```python
from build123d import *

# Parameters (mm, degrees)
SKETCH1_R           = 0.762
BOSS_EXTRUDE1_DEPTH = 0.381


with BuildPart() as part:
    # Sketch1 → Boss-Extrude1 (new, symmetric)
    with BuildSketch(Plane(origin=(0, 0, 0), x_dir=(1, 0, 0), z_dir=(0, 1, 0))):
        with BuildLine():
            Line((-0.172545192, 1.641958939), (1.605454808, 1.8288))
            Line((1.605454808, 1.8288), (7.828454808, 1.8288))
            ThreePointArc((7.828454808, 1.8288), (8.367270176, 1.605615367), (8.590454808, 1.0668))
            Line((8.590454808, 1.0668), (8.590454808, -1.0668))
            ThreePointArc((8.590454808, -1.0668), (8.367270176, -1.605615367), (7.828454808, -1.8288))
            Line((7.828454808, -1.8288), (1.605454808, -1.8288))
            Line((1.605454808, -1.8288), (-0.172545192, -1.641958939))
            ThreePointArc((-0.172545192, -1.641958939), (-1.651, 0), (-0.172545192, 1.641958939))
        make_face()
        with Locations(Location((0, 0, 0), (0, 0, 90))):
            Circle(SKETCH1_R, mode=Mode.SUBTRACT)
    extrude(amount=BOSS_EXTRUDE1_DEPTH, both=True)


solid = part.part
```
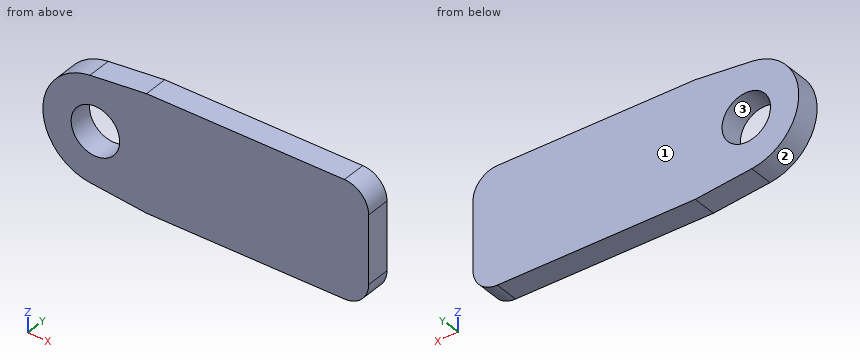
Here's how the part is built. I have some questions about the finished solid (model axes, mm). Face numbers are marked on the shaded views. Coordinates: 2 decimals unless noted, no trailing zeros. Order: outer loops, then holes, each group sorted by start corner. A loop starts at its lowest first (then second) coordinate and runs counter-clockwise, first axis right, second up. Notation, with made-up numbers: (82.25, -17.5) - (87.25, -17.5) arc R24 cw to (87.25, 10.5) - close; hole circle Ø4 at (-28.5, -30.5). An arc over 180 degrees is marked (long way). One line per question, with ' | ' between items.
(1) If I drill on L1, parallel to X at y = -0.15, z = -0.1; L2, parallel to X at y = 0.2, z = 0.3; L3, parallel to X at y = -0.15, z = -1.2, over which ranges is the centre line in solid material (lowest first)?
Report:
L1: x = -1.65 to -0.76, 0.76 to 8.59 | L2: x = -1.62 to -0.7, 0.7 to 8.59 | L3: x = -1.13 to 8.58
(2) Suppose I cut it at A-A on y = 0.15. List the corners of the cut face in (x, z) for me, and give its area (3 significant figures).
Report:
outline: (-0.17, -1.64) - (1.61, -1.83) - (7.83, -1.83) arc R0.76 ccw to (8.59, -1.07) - (8.59, 1.07) arc R0.76 ccw to (7.83, 1.83) - (1.61, 1.83) - (-0.17, 1.64) arc R1.65 ccw to start; hole circle Ø1.52 at (0, 0) | area: 33.4 mm2
(3) If we mould it in two halves opening along Z, with no side actions, what happens to the marked faces 1, 2 and 3? For each: pulls with the +Z half, pulls with the -Z half, needs draft (parallel to the pull), parting line crosses it, or undercut.
Report:
face 1: needs draft | face 2: parting line crosses it | face 3: undercut
(4) Suppose I cut it at B-B on z = -0.5. List the corners of the cut face in (x, y) for me, and give its area (3 significant figures).
Report:
outline: (-1.57, -0.38) - (-0.58, -0.38) - (-0.58, 0.38) - (-1.57, 0.38) - close; (0.58, -0.38) - (8.59, -0.38) - (8.59, 0.38) - (0.58, 0.38) - close | area: 6.87 mm2
(5) Suppose I cut it at D-D on z = -1.2. List the corners of the cut face in (x, y) for me, and give its area (3 significant figures).
Report:
outline: (-1.13, -0.38) - (8.58, -0.38) - (8.58, 0.38) - (-1.13, 0.38) - close | area: 7.40 mm2
(6) Suppose I cut it at C-C on x = 0.25. List the corners of the cut face in (y, z) for me.
Report:
outline: (-0.38, -1.69) - (0.38, -1.69) - (0.38, -0.72) - (-0.38, -0.72) - close; (-0.38, 0.72) - (0.38, 0.72) - (0.38, 1.69) - (-0.38, 1.69) - close
